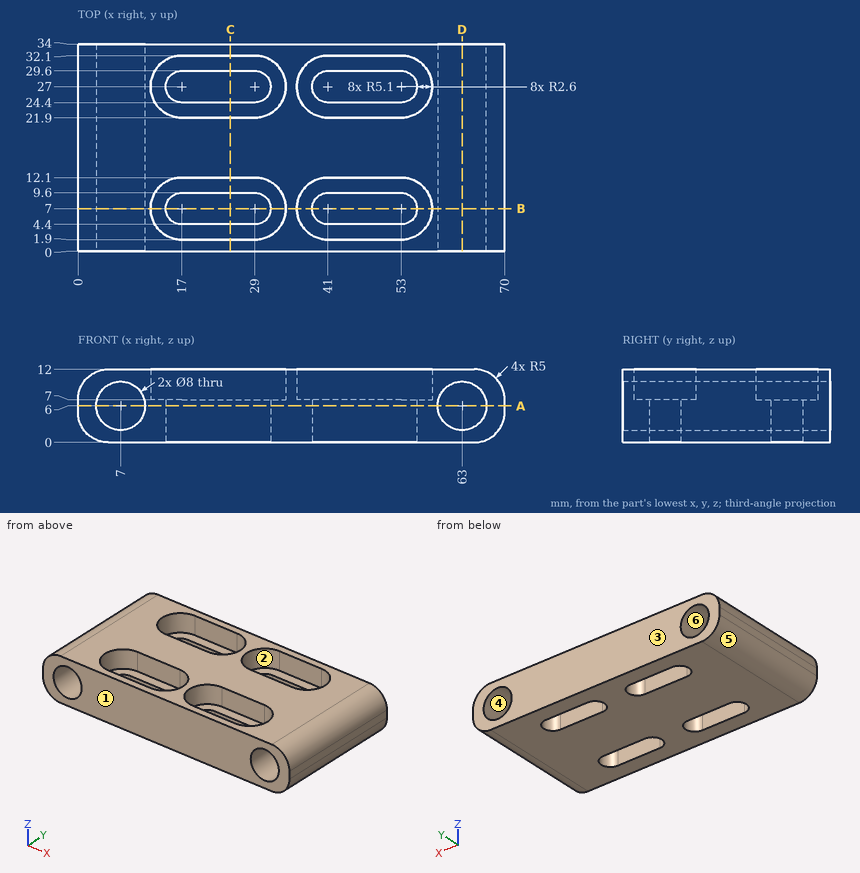
Drawing for the job (mm, zero at the part's lowest x, y, z). A direction names the side the tool comes from. Round coordinates to 2 decimals unless told otherwise and drop trailing zeros. Write each loop counter-clockwise with the first axis right and the second up, starting at its lowest first coordinate (ties: lowest second). Pieces come first, ordered by that corner, then holes.
Item 1: Band-saw the part on B-B on y = 7. Write the cut outline in (x, z), then the cut area to 3 significant figures.
Filled in:
outline: (0, 5) arc R5 ccw to (5, 0) - (14.4, 0) - (14.4, 7) - (11.9, 7) - (11.9, 12) - (5, 12) arc R5 ccw to (0, 7) - close; (31.6, 0) - (38.4, 0) - (38.4, 7) - (35.9, 7) - (35.9, 12) - (34.1, 12) - (34.1, 7) - (31.6, 7) - close; (55.6, 0) - (65, 0) arc R5 ccw to (70, 5) - (70, 7) arc R5 ccw to (65, 12) - (58.1, 12) - (58.1, 7) - (55.6, 7) - close; hole circle Ø8 at (7, 6); hole circle Ø8 at (63, 6)
area: 255 mm2
Item 2: Band-saw the part on D-D on x = 63. Write the cut outline in (y, z), then the cut area to 3 significant figures.
Filled in:
outline: (0, 0) - (34, 0) - (34, 2) - (0, 2) - close; (0, 10) - (34, 10) - (34, 12) - (0, 12) - close
area: 136 mm2
Item 3: Mould opens along Z. For the marked faces 3, 4, 5 and 6 say: released by +Z, released by -Z, zero draft, split by the parting line, or undercut.
Filled in:
face 3: zero draft
face 4: undercut
face 5: released by -Z
face 6: undercut
Item 4: Band-saw the part on C-C on x = 25. Write the cut outline in (y, z), then the cut area to 3 significant figures.
Filled in:
outline: (0, 0) - (4.4, 0) - (4.4, 7) - (1.9, 7) - (1.9, 12) - (0, 12) - close; (9.6, 0) - (24.4, 0) - (24.4, 7) - (21.9, 7) - (21.9, 12) - (12.1, 12) - (12.1, 7) - (9.6, 7) - close; (29.6, 0) - (34, 0) - (34, 12) - (32.1, 12) - (32.1, 7) - (29.6, 7) - close
area: 233 mm2
Item 5: Drop a flat-ended pin along its axis: pin 1 Ø8 at (x, y) = (18.5, 27.5) entering from +Z. Give the stop position or say it passes through.
Filled in:
pin 1: stops at z = 7
Item 6: Drill centre lines: L1, parallel to Y at x = 44, z = 10.5; L2, parallel to Y at x = 18, z = 0.5; L3, parallel to X at y = 21.5, z = 5.75. Where is each one in solid material? Low to high.
Filled in:
L1: y = 0 to 1.9, 12.1 to 21.9, 32.1 to 34
L2: y = 0 to 4.4, 9.6 to 24.4, 29.6 to 34
L3: x = 0 to 3.01, 10.99 to 59.01, 66.99 to 70
Item 7: Tool access for the marked faces 1 and 2: list every direction of +Z, -Z, +X, -X, +Y, -Y with a clear straight run to the whole face (end or side of a thin tool).
Filled in:
face 1: +Z, -Z, +X, -X, -Y
face 2: +Z
Item 8: Band-saw the part on A-A on z = 6. Write the cut outline in (x, y), then the cut area to 3 significant figures.
Filled in:
outline: (0, 0) - (3, 0) - (3, 34) - (0, 34) - close; (11, 0) - (59, 0) - (59, 34) - (11, 34) - close; (67, 0) - (70, 0) - (70, 34) - (67, 34) - close; hole (17, 4.4) - (29, 4.4) arc R2.6 ccw to (29, 9.6) - (17, 9.6) arc R2.6 ccw to start; hole (17, 24.4) - (29, 24.4) arc R2.6 ccw to (29, 29.6) - (17, 29.6) arc R2.6 ccw to start; hole (41, 4.4) - (53, 4.4) arc R2.6 ccw to (53, 9.6) - (41, 9.6) arc R2.6 ccw to start; hole (41, 24.4) - (53, 24.4) arc R2.6 ccw to (53, 29.6) - (41, 29.6) arc R2.6 ccw to start
area: 1,500 mm2
